Part model, mm, in its own coordinate system. Face numbers are marked on the shaded views. A direction names the side the tool comes from. Round coordinates to 2 decimals unless told otherwise and drop trailing zeros. Loops run counter-clockwise (first coordinate to the right, second up) from the corner with the lowest first, then second, coordinate; pieces in that order, holes last. Notation, with made-up numbers: M 41.5,35 L 71.5,35 A8 ccw 71.5,45 Z; hole C -32,68.5 d8. An arc over 180 degrees is marked long. Write each question's results on one line, items separated by ' | '.
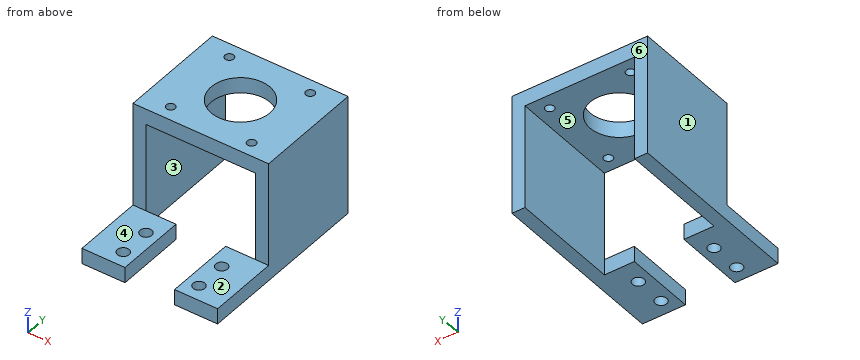
from build123d import *

# Parameters (mm, degrees)
EXTRUDE_START               = 40
SKETCH_1013_W               = 52
SKETCH_1013_H               = 42
EXTRUDE_1127_DEPTH          = 6
SKETCH_1179_W               = 5
SKETCH_1179_H               = 42
EXTRUDE_1393_DEPTH          = 40
SKETCH_1445_W               = 16.5
SKETCH_1445_H               = 27
EXTRUDE_1760_DEPTH          = 6
CUT_EXTRUDE_1818_DEPTH      = 72.38627319
CUT_EXTRUDE_1818_DEPTH_BACK = 72.38627319
SKETCH_1809_R               = 11.25
SKETCH_1809_R_2             = 1.7
CUT_EXTRUDE_1864_DEPTH      = 72.38627319
CUT_EXTRUDE_1864_DEPTH_BACK = 72.38627319
SKETCH_1856_R               = 2.25


with BuildPart() as part:
    # Sketch 1013 → Extrude 1127 (new body)
    with BuildSketch(Plane.XY.offset(EXTRUDE_START)):
        Rectangle(SKETCH_1013_W, SKETCH_1013_H)
    extrude(amount=EXTRUDE_1127_DEPTH)

    # Sketch 1179 → Extrude 1393 (add)
    with BuildSketch(Plane.XY):
        with Locations((-23.5, 0)):
            Rectangle(SKETCH_1179_W, SKETCH_1179_H)
        with Locations((23.5, 0)):
            Rectangle(SKETCH_1179_W, SKETCH_1179_H)
    extrude(amount=EXTRUDE_1393_DEPTH)

    # Sketch 1445 → Extrude 1760 (add)
    with BuildSketch(Plane.XY):
        with Locations((-17.75, -34.5)):
            Rectangle(SKETCH_1445_W, SKETCH_1445_H)
        with Locations((17.75, -34.5)):
            Rectangle(SKETCH_1445_W, SKETCH_1445_H)
    extrude(amount=EXTRUDE_1760_DEPTH)

    # Sketch 1809 → Cut-Extrude 1818 (cut, two sides: drawn at the far end of the back side and taken through both)
    with BuildSketch(Plane.XY.offset(-CUT_EXTRUDE_1818_DEPTH_BACK)):
        Circle(SKETCH_1809_R)
        with Locations((-15.5, -15.5)):
            Circle(SKETCH_1809_R_2)
        with Locations((-15.5, 15.5)):
            Circle(SKETCH_1809_R_2)
        with Locations((15.5, -15.5)):
            Circle(SKETCH_1809_R_2)
        with Locations((15.5, 15.5)):
            Circle(SKETCH_1809_R_2)
    extrude(amount=CUT_EXTRUDE_1818_DEPTH + CUT_EXTRUDE_1818_DEPTH_BACK, mode=Mode.SUBTRACT)

    # Sketch 1856 → Cut-Extrude 1864 (cut, two sides: drawn at the far end of the back side and taken through both)
    with BuildSketch(Plane.XY.offset(-CUT_EXTRUDE_1864_DEPTH_BACK)):
        with Locations((-14.5, -30)):
            Circle(SKETCH_1856_R)
        with Locations((-14.5, -42)):
            Circle(SKETCH_1856_R)
        with Locations((14.5, -30)):
            Circle(SKETCH_1856_R)
        with Locations((14.5, -42)):
            Circle(SKETCH_1856_R)
    extrude(amount=CUT_EXTRUDE_1864_DEPTH + CUT_EXTRUDE_1864_DEPTH_BACK, mode=Mode.SUBTRACT)


solid = part.part
Item 1: Drop flat-ended pins along their axis: P1, Ø3.5, axis at x = 14.5, y = -30, coming from the -Z side; P2, Ø12, axis at x = -13, z = 39.5, coming from the -Y side; P3, Ø5, axis at x = -15, y = -38.5, coming from the +Z side; P4, Ø5, axis at x = 13, z = 2, coming from the +Y side. Give the stop position or say it passes through.
Filled sheet:
P1: through | P2: y = -21 | P3: z = 6 | P4: y = -21
Item 2: Band-saw the part on B-B on x = -19.5. Give the cut face in (y, z).
Filled sheet:
outline: M -48,0 L -21,0 L -21,6 L -48,6 Z; M -21,40 L 21,40 L 21,46 L -21,46 Z
Item 3: Wall check: L1, parallel to X at y = -42, z = 3; L2, parallel to Y at x = -15.5, z = 43.15; L3, parallel to X at y = -15.5, z = 42.55. Give the ranges that are in metal, low to high.
Filled sheet:
L1: -26 to -16.75, -12.25 to -9.5, 9.5 to 12.25, 16.75 to 26 | L2: -21 to -17.2, -13.8 to 13.8, 17.2 to 21 | L3: -26 to -17.2, -13.8 to 13.8, 17.2 to 26
Item 4: Band-saw the part on D-D on z = 33. Give the cut face in (x, y), and give its area (3 significant figures).
Filled sheet:
outline: M -26,-21 L -21,-21 L -21,21 L -26,21 Z; M 21,-21 L 26,-21 L 26,21 L 21,21 Z | area: 420 mm^2
Item 5: Band-saw the part on A-A on z = 3. Give the cut face in (x, y).
Filled sheet:
outline: M -26,-48 L -9.5,-48 L -9.5,-21 L -21,-21 L -21,21 L -26,21 Z; M 9.5,-48 L 26,-48 L 26,21 L 21,21 L 21,-21 L 9.5,-21 Z; hole C -14.5,-42 d4.5; hole C -14.5,-30 d4.5; hole C 14.5,-42 d4.5; hole C 14.5,-30 d4.5
Item 6: Which spindle directions (+Z, -Z, +X, -X, +Y, -Y) get a long thin tool onto all of the face, cutting with end or side? Do the marked faces 4, 5 and 6. Say none if no direction does.
Filled sheet:
face 4: +Z, +X, -X, -Y | face 5: -Z, +Y, -Y | face 6: +Z, -Z, +X, -X, +Y
Item 7: Two-plate mould, pull along X, no slides. Class the marked faces 1, 2 and 3: +X half, -X half, draft (parallel to the pull), parting line (faces both ways), or undercut.
Filled sheet:
face 1: -X half | face 2: draft | face 3: undercut
Item 8: Band-saw the part on C-C on y = -30. Give the cut face in (x, z), and give its area (3 significant figures).
Filled sheet:
outline: M -26,0 L -16.75,0 L -16.75,6 L -26,6 Z; M -12.25,0 L -9.5,0 L -9.5,6 L -12.25,6 Z; M 9.5,0 L 12.25,0 L 12.25,6 L 9.5,6 Z; M 16.75,0 L 26,0 L 26,6 L 16.75,6 Z | area: 144 mm^2
